Autodesk Inventor part; units mm, degrees
ref_plane "Work Plane1" through (0, 2.5, 0) normal (0, 1, 0) x (1, 0, 0)
ref_plane "YZ Plane" through (0, 0, 0) normal (1, 0, 0) x (0, 1, 0)
ref_plane "XZ Plane" through (0, 0, 0) normal (0, 1, 0) x (-1, 0, 0)
sketch "Sketch1" plane through (0, 0, 0) normal (0, 1, 0) x (-1, 0, 0)
  circle A0 centre (0, 0) radius 7
  circle A1 centre (0, 0) radius 2.5
  dimension "d0" = 14
  dimension "d1" = 5
extrude "Extrusion1" add sketch "Sketch1" along normal blind 5
sketch "Sketch2" plane through (0, 5, 0) normal (0, 1, 0) x (1, 0, 0)
  circle A0 centre (0, 0) radius 7
  circle A1 centre (0, 0) radius 2.5
  circle A2 centre (0, 0) radius 3
  circle A3 centre (0, 0) radius 6
  dimension "d4" = 6
  dimension "d5" = 1
extrude "Extrusion2" cut sketch "Sketch2" against normal blind 1 contours A3
ref_plane "Work Plane1" through (0, 2.5, 0) normal (0, 1, 0) x (1, 0, 0)
mirror "Mirror1" about plane through (0, 2.5, 0) normal (0, 1, 0) of "Extrusion2"
properties part number "Bearing5X15X5"
Model file for the job. Use its own axes, mm. A direction names the side the tool comes from. Coordinates: 2 decimals unless noted, no trailing zeros. Write each loop counter-clockwise with the first axis right and the second up, starting at its lowest first coordinate (ties: lowest second). Pieces come first, ordered by that corner, then holes. Notation, with made-up numbers: (-32.75, -14) - (-8.75, -14) arc R24 ccw to (-8.75, 25) - close; hole circle Ø1 at (1, 80). An arc over 180 degrees is marked (long way). Use a Markdown table: item, result. Add a question column.
Item 1: Band-saw the part on A-A, the plane x = 0. Write the cut outline in (y, z), and give its area (3 significant figures).
Item 2: Band-saw the part on D-D, the plane y = 3.6. Write the cut outline in (x, z), and give its area (3 significant figures).
Item 3: Band-saw the part on C-C, the plane y = 4.35. Write the cut outline in (x, z).
Item 4: 3-axis set-ups, long thin cutter, end or side, ignore diameter. For faces 4 (the face through (3, 1, 1)), 5 (the face through (-3, 4.5, -0.1)), 6 (the face through (-6, 0, 2)): which of +Z, -Z, +X, -X, +Y, -Y reach the whole face in a straight line?
Item 5: Drop flat-ended pins along their axis: pin 1 (1 mm diameter, centred on x = -4, z = 1, fed in from +Y); pin 2 (3.5 mm diameter, centred on x = 2.5, z = -2.5, fed in from -Y); pin 3 (1.5 mm diameter, centred on x = 2, y = 2.5, fed in from -Z); pin 4 (3 mm diameter, centred on x = -5.5, y = 3.5, fed in from +Z). Give the stop position or say it passes through.
Item 6: Band-saw the part on B-B, the plane z = 0. Write the cut outline in (x, y).
Item 7: Drill centre lines: line 1 along Z through (x, y) = (0, 4.25); line 2 along Z through (x, y) = (-1, 0.25); line 3 along Y through (x, z) = (1.25, -5.5). Where is each one in solid material? Low to high.
Item 8: Two-plate mould, pull along Z, no slides. Class faces 1 (the face through (-3, 4, 1)), 2 (the face through (2, 5, 2)), 3 (the face through (-6.466, 2.465, 2.681)): pulls with the +Z half, pulls with the -Z half, needs draft (parallel to the pull), parting line crosses it, or undercut.
A:
| question | item | result |
|---|---|---|
| 1 | outline | (0, -7) - (5, -7) - (5, -6) - (4, -6) - (4, -3) - (5, -3) - (5, -2.5) - (0, -2.5) - (0, -3) - (1, -3) - (1, -6) - (0, -6) - close; (0, 2.5) - (5, 2.5) - (5, 3) - (4, 3) - (4, 6) - (5, 6) - (5, 7) - (0, 7) - (0, 6) - (1, 6) - (1, 3) - (0, 3) - close |
| 1 | area | 33.0 mm² |
| 2 | outline | circle Ø14 at (0, 0); hole circle Ø5 at (0, 0) |
| 2 | area | 134 mm² |
| 3 | outline | circle Ø14 at (0, 0); circle Ø6 at (0, 0); hole circle Ø12 at (0, 0); hole circle Ø5 at (0, 0) |
| 4 | face 4 | -Y |
| 4 | face 5 | +Y |
| 4 | face 6 | +Z, -Z, +X, -X, -Y |
| 5 | pin 1 | stops at y = 4 |
| 5 | pin 2 | stops at y = 0 |
| 5 | pin 3 | stops at z = -6.89 |
| 5 | pin 4 | stops at z = 5.74 |
| 6 | outline | (-7, 0) - (-6, 0) - (-6, 1) - (-3, 1) - (-3, 0) - (-2.5, 0) - (-2.5, 5) - (-3, 5) - (-3, 4) - (-6, 4) - (-6, 5) - (-7, 5) - close; (2.5, 0) - (3, 0) - (3, 1) - (6, 1) - (6, 0) - (7, 0) - (7, 5) - (6, 5) - (6, 4) - (3, 4) - (3, 5) - (2.5, 5) - close |
| 7 | line 1 | z = -7 to -6, -3 to -2.5, 2.5 to 3, 6 to 7 |
| 7 | line 2 | z = -6.93 to -5.92, -2.83 to -2.29, 2.29 to 2.83, 5.92 to 6.93 |
| 7 | line 3 | y = 1 to 4 |
| 8 | face 1 | undercut |
| 8 | face 2 | needs draft |
| 8 | face 3 | parting line crosses it |
